from build123d import *

# Parameters (mm, degrees)
F0_R     = 0.75
F0_R_2   = 0.5
F2_DEPTH = 15
F3_DEPTH = 10


with BuildPart() as f2:
    # F0 (on Top) → F2 (new body)
    with BuildSketch(Plane.XY):
        Polygon((0.5, 3), (0, 0), (0.5, 0), (0.5, 0.5), align=None)
        with BuildLine():
            Line((0.5, 0), (0, 0))
            Line((0, 0), (0, -1.5))
            ThreePointArc((0, -1.5), (1.5, -3), (3, -1.5))
            Line((3, -1.5), (3, 0))
            Line((3, 0), (1.5, 0))
            Line((1.5, 0), (1.4034414795, 0))
            Line((1.4034414795, 0), (0.5, 0))
        make_face()
        with Locations((1.5, -1.5)):
            Circle(F0_R, mode=Mode.SUBTRACT)
        Polygon((0.5, 0.5), (0.5, 0), (1.4034414795, 0), (1.5, 0), (3, 0), (7, 0), (8.5, 0), (9.5, 0), (9.5, 0.5), align=None)
        Polygon((4.9166666667, 29.5), (0.5, 3), (0.5, 0.5), (1.4948575599, 6.9113042752), (1.6500299737, 7.9113042752), (1.8052023875, 8.9113042752), (2.6836806371, 14.5726085504), (2.8000599475, 15.3226085504), (2.9164392578, 16.0726085504), (3.9112968178, 22.4839128256), (3.9500899212, 22.7339128256), (3.9888830247, 22.9839128256), (5, 29.5), align=None)
        Polygon((5, 30), (4.9166666667, 29.5), (5, 29.5), (5.0833333333, 29.5), align=None)
        Polygon((9.5, 3), (9.5, 0.5), (9.5, 0), (10, 0), align=None)
        Polygon((8.5051424401, 6.9113042752), (9.5, 0.5), (9.5, 3), (5.0833333333, 29.5), (5, 29.5), (6.0111169753, 22.9839128256), (6.0499100788, 22.7339128256), (6.0887031822, 22.4839128256), (7.0835607422, 16.0726085504), (7.1999400525, 15.3226085504), (7.3163193629, 14.5726085504), (8.1947976125, 8.9113042752), align=None)
        with BuildLine():
            Line((10, 0), (9.5, 0))
            Line((9.5, 0), (8.5, 0))
            Line((8.5, 0), (7, 0))
            Line((7, 0), (7, -1.5))
            ThreePointArc((7, -1.5), (8.5, -3), (10, -1.5))
            Line((10, -1.5), (10, 0))
        make_face()
        with Locations((8.5, -1.5)):
            Circle(F0_R, mode=Mode.SUBTRACT)
        with BuildLine():
            Line((1.6500299737, 7.9113042752), (1.4948575599, 6.9113042752))
            Line((1.4948575599, 6.9113042752), (2.6500299737, 6.9113042752))
            ThreePointArc((2.6500299737, 6.9113042752), (3.6500299737, 7.9113042752), (2.6500299737, 8.9113042752))
            Line((2.6500299737, 8.9113042752), (1.8052023875, 8.9113042752))
            Line((1.8052023875, 8.9113042752), (1.6500299737, 7.9113042752))
        make_face()
        with BuildLine():
            ThreePointArc((2.6500299737, 7.4113042752), (2.2964765831, 8.2648576658), (3.1500299737, 7.9113042752))
            ThreePointArc((3.1500299737, 7.9113042752), (3.0035833643, 7.5577508846), (2.6500299737, 7.4113042752))
        make_face(mode=Mode.SUBTRACT)
        with BuildLine():
            Line((7.3499700263, 6.9113042752), (8.5051424401, 6.9113042752))
            Line((8.5051424401, 6.9113042752), (8.1947976125, 8.9113042752))
            Line((8.1947976125, 8.9113042752), (7.3499700263, 8.9113042752))
            ThreePointArc((7.3499700263, 8.9113042752), (6.3499700263, 7.9113042752), (7.3499700263, 6.9113042752))
        make_face()
        with Locations((7.3499700263, 7.9113042752)):
            Circle(F0_R_2, mode=Mode.SUBTRACT)
        with BuildLine():
            Line((2.8000599475, 15.3226085504), (2.6836806371, 14.5726085504))
            Line((2.6836806371, 14.5726085504), (3.5500599475, 14.5726085504))
            Line((3.5500599475, 14.5726085504), (3.5500599475, 14.8226085504))
            ThreePointArc((3.5500599475, 14.8226085504), (3.1965065569, 14.9690551598), (3.0500599475, 15.3226085504))
            Line((3.0500599475, 15.3226085504), (2.8000599475, 15.3226085504))
        make_face()
        with BuildLine():
            Line((3.5500599475, 14.8226085504), (3.5500599475, 14.5726085504))
            ThreePointArc((3.5500599475, 14.5726085504), (4.0803900334, 14.7922784645), (4.3000599475, 15.3226085504))
            Line((4.3000599475, 15.3226085504), (4.0500599475, 15.3226085504))
            ThreePointArc((4.0500599475, 15.3226085504), (3.9036133381, 14.9690551598), (3.5500599475, 14.8226085504))
        make_face()
        with BuildLine():
            Line((4.0500599475, 15.3226085504), (4.3000599475, 15.3226085504))
            ThreePointArc((4.3000599475, 15.3226085504), (4.0803900334, 15.8529386363), (3.5500599475, 16.0726085504))
            Line((3.5500599475, 16.0726085504), (3.5500599475, 15.8226085504))
            ThreePointArc((3.5500599475, 15.8226085504), (3.9036133381, 15.676161941), (4.0500599475, 15.3226085504))
        make_face()
        with BuildLine():
            Line((2.9164392578, 16.0726085504), (2.8000599475, 15.3226085504))
            Line((2.8000599475, 15.3226085504), (3.0500599475, 15.3226085504))
            ThreePointArc((3.0500599475, 15.3226085504), (3.1965065569, 15.676161941), (3.5500599475, 15.8226085504))
            Line((3.5500599475, 15.8226085504), (3.5500599475, 16.0726085504))
            Line((3.5500599475, 16.0726085504), (2.9164392578, 16.0726085504))
        make_face()
        with BuildLine():
            Line((6.9499400525, 15.3226085504), (7.1999400525, 15.3226085504))
            Line((7.1999400525, 15.3226085504), (7.0835607422, 16.0726085504))
            Line((7.0835607422, 16.0726085504), (6.4499400525, 16.0726085504))
            ThreePointArc((6.4499400525, 16.0726085504), (5.9196099666, 15.8529386363), (5.6999400525, 15.3226085504))
            Line((5.6999400525, 15.3226085504), (5.9499400525, 15.3226085504))
            ThreePointArc((5.9499400525, 15.3226085504), (6.4499400525, 15.8226085504), (6.9499400525, 15.3226085504))
        make_face()
        with BuildLine():
            Line((6.4499400525, 14.5726085504), (7.3163193629, 14.5726085504))
            Line((7.3163193629, 14.5726085504), (7.1999400525, 15.3226085504))
            Line((7.1999400525, 15.3226085504), (6.9499400525, 15.3226085504))
            ThreePointArc((6.9499400525, 15.3226085504), (6.4499400525, 14.8226085504), (5.9499400525, 15.3226085504))
            Line((5.9499400525, 15.3226085504), (5.6999400525, 15.3226085504))
            ThreePointArc((5.6999400525, 15.3226085504), (5.9196099666, 14.7922784645), (6.4499400525, 14.5726085504))
        make_face()
        with BuildLine():
            Line((4.0750899212, 22.7339128256), (3.9500899212, 22.7339128256))
            Line((3.9500899212, 22.7339128256), (3.9112968178, 22.4839128256))
            Line((3.9112968178, 22.4839128256), (4.2000899212, 22.4839128256))
            Line((4.2000899212, 22.4839128256), (4.2000899212, 22.6089128256))
            ThreePointArc((4.2000899212, 22.6089128256), (4.1117015736, 22.6455244779), (4.0750899212, 22.7339128256))
        make_face()
        with BuildLine():
            ThreePointArc((4.2000899212, 22.4839128256), (4.3768666165, 22.5571361303), (4.4500899212, 22.7339128256))
            Line((4.4500899212, 22.7339128256), (4.3250899212, 22.7339128256))
            ThreePointArc((4.3250899212, 22.7339128256), (4.2884782689, 22.6455244779), (4.2000899212, 22.6089128256))
            Line((4.2000899212, 22.6089128256), (4.2000899212, 22.4839128256))
        make_face()
        with BuildLine():
            ThreePointArc((4.4500899212, 22.7339128256), (4.3768666165, 22.9106895209), (4.2000899212, 22.9839128256))
            Line((4.2000899212, 22.9839128256), (4.2000899212, 22.8589128256))
            ThreePointArc((4.2000899212, 22.8589128256), (4.2884782689, 22.8223011732), (4.3250899212, 22.7339128256))
            Line((4.3250899212, 22.7339128256), (4.4500899212, 22.7339128256))
        make_face()
        with BuildLine():
            Line((4.2000899212, 22.9839128256), (3.9888830247, 22.9839128256))
            Line((3.9888830247, 22.9839128256), (3.9500899212, 22.7339128256))
            Line((3.9500899212, 22.7339128256), (4.0750899212, 22.7339128256))
            ThreePointArc((4.0750899212, 22.7339128256), (4.1117015736, 22.8223011732), (4.2000899212, 22.8589128256))
            Line((4.2000899212, 22.8589128256), (4.2000899212, 22.9839128256))
        make_face()
        with BuildLine():
            Line((6.0499100788, 22.7339128256), (6.0111169753, 22.9839128256))
            Line((6.0111169753, 22.9839128256), (5.7999100788, 22.9839128256))
            ThreePointArc((5.7999100788, 22.9839128256), (5.6231333835, 22.9106895209), (5.5499100788, 22.7339128256))
            Line((5.5499100788, 22.7339128256), (5.6749100788, 22.7339128256))
            ThreePointArc((5.6749100788, 22.7339128256), (5.7999100788, 22.8589128256), (5.9249100788, 22.7339128256))
            Line((5.9249100788, 22.7339128256), (6.0499100788, 22.7339128256))
        make_face()
        with BuildLine():
            Line((6.0887031822, 22.4839128256), (6.0499100788, 22.7339128256))
            Line((6.0499100788, 22.7339128256), (5.9249100788, 22.7339128256))
            ThreePointArc((5.9249100788, 22.7339128256), (5.7999100788, 22.6089128256), (5.6749100788, 22.7339128256))
            Line((5.6749100788, 22.7339128256), (5.5499100788, 22.7339128256))
            ThreePointArc((5.5499100788, 22.7339128256), (5.6231333835, 22.5571361303), (5.7999100788, 22.4839128256))
            Line((5.7999100788, 22.4839128256), (6.0887031822, 22.4839128256))
        make_face()
    extrude(amount=F2_DEPTH)

    # F1 (on Right) → F3 (cut)
    with BuildSketch(Plane.YZ):
        Polygon((-3, 2.5), (0, 2.5), (0, 7.5), (0, 12.5), (-3, 12.5), align=None)
    extrude(amount=F3_DEPTH, mode=Mode.SUBTRACT)


solid = f2.part
For this review, take the finished solid that the model builds, in its own axes (mm). A direction names the side the tool comes from. Round coordinates to 2 decimals unless told otherwise and drop trailing zeros. Loops run counter-clockwise (first coordinate to the right, second up) from the corner with the lowest first, then second, coordinate; pieces in that order, holes last. Notation, with made-up numbers: (0, 13) - (13, 13) arc R27 ccw to (13, 38) - close; hole circle Ø6 at (56.25, 49.25). An arc over 180 degrees is marked (long way). Put each result on its own line as item: value. Start each with the question number.
1. Consider section A-A on y = 19.5. State the section outline as (x, z) points, plus the area to 3 significant figures.
2. Consider section C-C on y = 10.5. State the section outline as (x, z) points, plus the area to 3 significant figures.
3. Mouldability with a two-part tool opening along Y and no side actions: class faces 1 (the flat face through (7, -1, 14)), 2 (the cylindrical face through (1.5, -3, 1.2)), 3 (the flat face through (2.238, 11.702, 7.395)) as +Y half, -Y half, draft (parallel to the pull), parting line (faces both ways), or undercut.
4. Consider section B-B on z = 8. State how many separate pieces and enclosed holes the cut face has, plus the area to 3 significant figures.
5. Insertion check: P1, Ø0.9, axis at x = 8, z = 8.5, coming from the -Y side; P2, Ø3, axis at y = 8.5, z = 9.5, coming from the -X side; P3, Ø1, axis at y = 21, z = 11, coming from the -X side. Each pin has a flat end and moves straight along its axis. Give the tip position at first contact, or say it passes through.
6. For probe 1 along X at (y, z) = (-1.5, 1.2); probe 2 along X at (y, z) = (3, 3.5); probe 3 along X at (y, z) = (5, 8.5), list the stretches that pass through material, from the lowest coordinate up. Write a range as [from, to].
7. For faces 4 (the flat face through (3, -1, 14)), 5 (the flat face through (10, -1, 14)), 6 (the cylindrical face through (6.35, 7.93, 7.4)), list the 3-axis set-ups (+Z, -Z, +X, -X, +Y, -Y) from which the entire face can be reached by the end or side of a thin tool; tool diameter is ignored.
Result sheet:
1. outline: (3.25, 0) - (3.45, 0) - (3.45, 15) - (3.25, 15) - close; (6.55, 0) - (6.75, 0) - (6.75, 15) - (6.55, 15) - close
1. area: 5.95 mm^2
2. outline: (1.75, 0) - (2.05, 0) - (2.05, 15) - (1.75, 15) - close; (7.95, 0) - (8.25, 0) - (8.25, 15) - (7.95, 15) - close
2. area: 9.05 mm^2
3. face 1: draft
3. face 2: -Y half
3. face 3: undercut
4. separate pieces: 1
4. enclosed holes: 7
4. area: 27.9 mm^2
5. P1: y = 0
5. P2: x = 1.17
5. P3: x = 3.42
6. probe 1: [0, 0.75], [2.25, 3], [7, 7.75], [9.25, 10]
6. probe 2: [0.5, 0.89], [9.11, 9.5]
6. probe 3: [0.83, 1.2], [8.8, 9.17]
7. face 4: +Z, -Z, -Y
7. face 5: +Z, -Z, +X, +Y, -Y
7. face 6: +Z, -Z
